The drawing under review shows one solid part. Ordinate dimensions are in mm from its lowest x, y, z. Round coordinates to 2 decimals unless told otherwise and drop trailing zeros. Order: outer loops, then holes, each group sorted by start corner. A loop starts at its lowest first (then second) coordinate and runs counter-clockwise, first axis right, second up. Notation, with made-up numbers: M 56,3.5 L 82,3.5 A30 ccw 82,34.5 Z; hole C 16,33 d7. An arc over 180 degrees is marked long. Use a Markdown table: item, result.
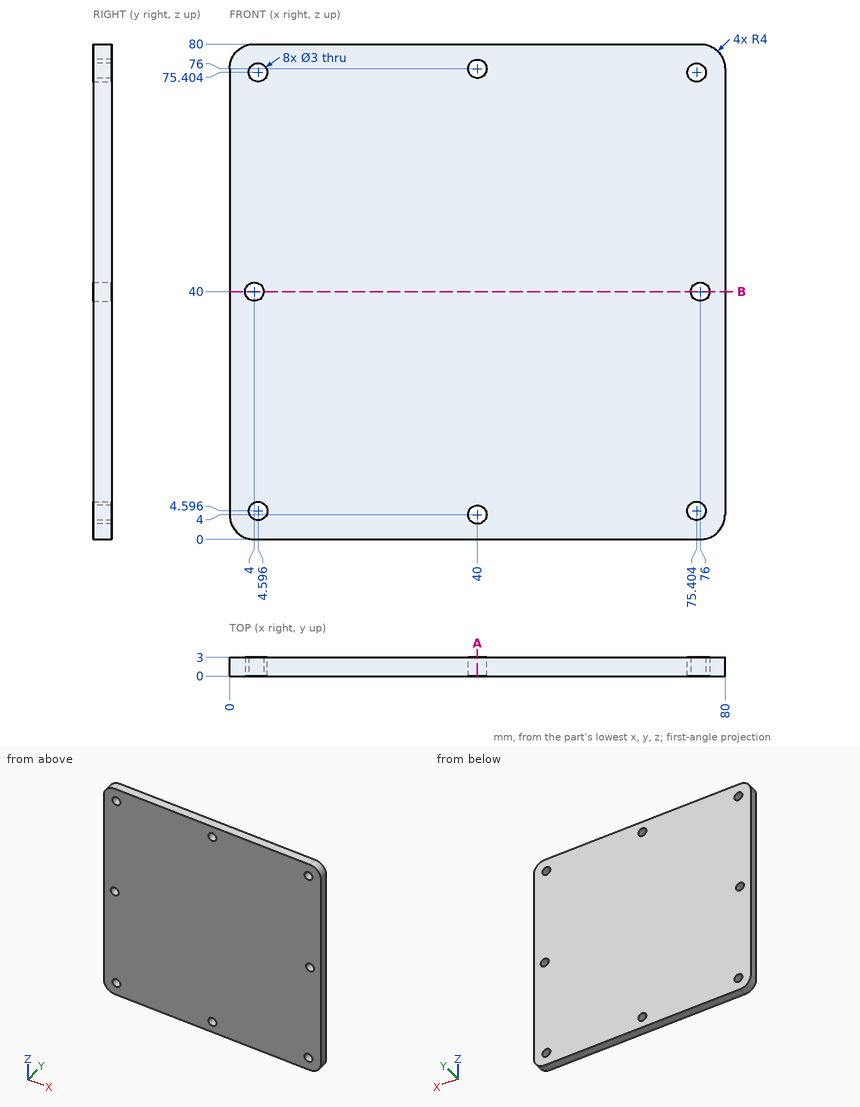
Q1. Wall thickness on line 1 along Z through (x, y) = (40, 0.9); line 2 along Z through (x, y) = (41, 1.3); line 3 along Z through (x, y) = (76, 2.45): over which ranges is each line inside the solid? List them lowest first. Write a range as [from, to].
Determined:
| item | result |
|---|---|
| line 1 | z = [0, 2.5], [5.5, 74.5], [77.5, 80] |
| line 2 | z = [0, 2.88], [5.12, 74.88], [77.12, 80] |
| line 3 | z = [0, 3.22], [5.97, 38.5], [41.5, 74.03], [76.78, 80] |
Q2. Add section B-B (z = 40). Write out the cut boundary in (x, y), then the cut area to 3 significant figures.
Determined:
| item | result |
|---|---|
| outline | M 0,0 L 2.5,0 L 2.5,3 L 0,3 Z; M 5.5,0 L 74.5,0 L 74.5,3 L 5.5,3 Z; M 77.5,0 L 80,0 L 80,3 L 77.5,3 Z |
| area | 222 mm^2 |
Q3. Add section A-A (x = 40). Write out the cut boundary in (y, z).
Determined:
| item | result |
|---|---|
| outline | M 0,0 L 3,0 L 3,2.5 L 0,2.5 Z; M 0,5.5 L 3,5.5 L 3,74.5 L 0,74.5 Z; M 0,77.5 L 3,77.5 L 3,80 L 0,80 Z |
